Here's how the part is built. I have some questions about the finished solid (model axes, mm). Face numbers are marked on the shaded views. A direction names the side the tool comes from. Give positions to 0.01 mm unless a question says otherwise; leave off trailing zeros. Write each loop counter-clockwise with the first axis right and the second up, starting at its lowest first coordinate (ties: lowest second). Pieces come first, ordered by that corner, then holes. Notation, with made-up numbers: (83, 86) - (112, 86) arc R18 cw to (112, 90) - close; hole circle Ø8 at (40.5, 58). An arc over 180 degrees is marked (long way). Use a Markdown table: item, result.
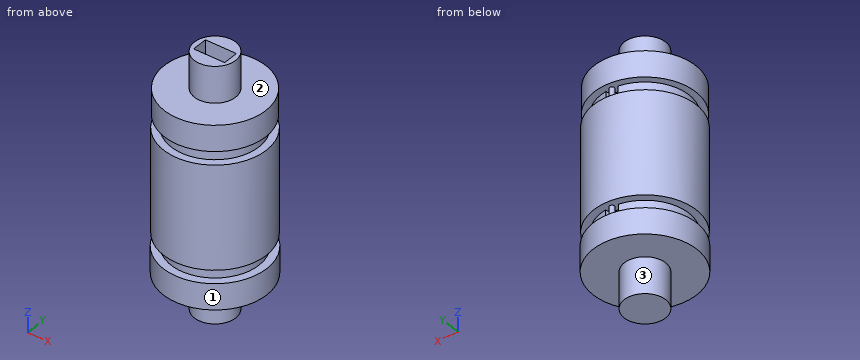
Autodesk Inventor part; units mm, degrees
ref_plane "YZ Plane" through (0, 0, 0) normal (1, 0, 0) x (0, 1, 0)
ref_plane "XZ Plane" through (0, 0, 0) normal (0, 1, 0) x (-1, 0, 0)
ref_plane "XY Plane" through (0, 0, 0) normal (0, 0, 1) x (1, 0, 0)
sketch "Sketch1" plane through (0, 0, 0) normal (0, 0, 1) x (1, 0, 0)
  circle A0 centre (0, 0) radius 10
  dimension "d0" = 20
extrude "Extrusion1" add sketch "Sketch1" along normal blind 5
sketch "Sketch2" plane through (0, 0, 5) normal (0, 0, 1) x (1, 0, 0)
  circle A0 centre (0, 0) radius 8.5
  circle A1 centre (-6.4588, 5.5258) radius 1.5
  dimension "d3" = 17
  dimension "d4" = 3
extrude "Extrusion2" add sketch "Sketch2" along normal blind 2.5 contours A0 A1 | A1 A0 picked at (2.8228, -1.7231) picked at (-6.0787, 5.1859)
sketch "Sketch3" plane through (0, 0, 7.5) normal (0, 0, 1) x (1, 0, 0)
  circle A0 centre (0, 0) radius 8.5
  circle A1 centre (0, 8.5) radius 1.25
  dimension "d7" = 2.5
extrude "Extrusion3" cut sketch "Sketch3" against normal blind 2.5 contours A1 A0 | A0 A1 picked at (0, 8.0765) picked at (0.0361, 8.9083)
sketch "Sketch4" plane through (0, 0, 7.5) normal (0, 0, 1) x (1, 0, 0)
  line L0 (-1.2337, 8.4081) -> (1.2466, 8.4081)
  circle A0 centre (0.0064, 8.4081) radius 0.5
  circle A1 centre (0, 0) radius 10
  dimension "d10" = 8.4081
  dimension "d11" = 1
extrude "Extrusion4" add sketch "Sketch4" against normal blind 2.5 contours A0 L0 | L0 A0
sketch "Sketch5" plane through (0, 0, 7.5) normal (0, 0, 1) x (1, 0, 0)
  circle A0 centre (0, 0) radius 9.9248
extrude "Extrusion5" add sketch "Sketch5" along normal blind 20
sketch "Sketch6" plane through (0, 0, 27.5) normal (0, 0, 1) x (1, 0, 0)
  circle A0 centre (0, 0) radius 8.5
extrude "Extrusion6" add sketch "Sketch6" along normal blind 2.5
sketch "Sketch7" plane through (0, 0, 30) normal (0, 0, 1) x (1, 0, 0)
  circle A0 centre (0.0064, 8.4081) radius 0.5
  circle A1 centre (0.0064, 8.4081) radius 0.5
  circle A2 centre (0.0064, 8.4081) radius 1.1746
  point P0 (0, 0)
extrude "Extrusion7" cut sketch "Sketch7" against normal blind 2.5 contours A0 | A2
sketch "Sketch8" plane through (0, 0, 30) normal (0, 0, 1) x (1, 0, 0)
  circle A0 centre (0.0064, 8.4081) radius 0.5
  circle A1 centre (0.0064, 8.4081) radius 0.5
  point P0 (0, 0)
extrude "Extrusion8" add sketch "Sketch8" against normal blind 2.5
sketch "Sketch9" plane through (0, 0, 30) normal (0, 0, 1) x (1, 0, 0)
  circle A0 centre (0, 0) radius 9.8132
extrude "Extrusion9" add sketch "Sketch9" along normal blind 5
sketch "Sketch10" plane through (0, 0, 35) normal (0, 0, 1) x (1, 0, 0)
  circle A0 centre (0, 0) radius 4
  line L0 (-3, 1.5) -> (3, 1.5)
  line L1 (3, 1.5) -> (3, -1.5)
  line L2 (3, -1.5) -> (-3, -1.5)
  line L3 (-3, -1.5) -> (-3, 1.5)
  dimension "d24" = 8
  dimension "d25" = 6
  dimension "d26" = 3
  dimension "d27" = 1.5
  dimension "d28" = 3
extrude "Extrusion10" add sketch "Sketch10" along normal blind 7
sketch "Sketch11" plane through (0, 0, 0) normal (0, 0, -1) x (-1, 0, 0)
  circle A0 centre (0, 0) radius 4
  dimension "d31" = 8
extrude "Extrusion11" add sketch "Sketch11" along normal blind 7
properties part number "Roller"
Item 1: For the marked faces 1, 2 and 3, which set-ups out of +Z, -Z, +X, -X, +Y, -Y let a thin tool reach every point of the face, with its end or its side?
Values:
| item | result |
|---|---|
| face 1 | +Z, -Z |
| face 2 | +Z |
| face 3 | -Z |
Item 2: If we section it at B-B, the plane z = 38: Write out the boundary of the cut face in (x, y).
Values:
| item | result |
|---|---|
| outline | circle Ø8 at (0, 0); hole (-3, -1.5) - (3, -1.5) - (3, 1.5) - (-3, 1.5) - close |
Item 3: Will these pins go through, and if not, where does the flat tip stop? pin 1 Ø4 at (x, z) = (-1.5, 36) entering from +Y; pin 2 Ø1.5 at (x, z) = (2.5, 33) entering from +Y; pin 3 Ø3.5 at (y, z) = (0.5, 38) entering from -X.
Values:
| item | result |
|---|---|
| pin 1 | stops at y = 9.81 |
| pin 2 | stops at y = 9.66 |
| pin 3 | stops at x = -4 |
Item 4: I need wall thicknesses on line 1 along Z through (x, y) = (-6.75, 6.75); line 2 along X through (y, z) = (-0.25, 28); line 3 along Z through (x, y) = (-4.25, -3). Which ranges of each line are inside material? Lowest first, please. Write a range as [from, to].
Values:
| item | result |
|---|---|
| line 1 | z = [0, 5], [7.5, 27.5], [30, 35] |
| line 2 | x = [-8.5, 8.5] |
| line 3 | z = [0, 35] |
Item 5: If we section it at D-D, the plane z = 24: Write out the boundary of the cut face in (x, y), plus the area to 3 significant figures.
Values:
| item | result |
|---|---|
| outline | circle Ø19.85 at (0, 0) |
| area | 309 mm2 |
Item 6: If we section it at C-C, the plane x = 5: Write out the boundary of the cut face in (y, z).
Values:
| item | result |
|---|---|
| outline | (-8.66, 0) - (8.66, 0) - (8.66, 5) - (6.87, 5) - (6.87, 7.5) - (8.57, 7.5) - (8.57, 27.5) - (6.87, 27.5) - (6.87, 30) - (8.44, 30) - (8.44, 35) - (-8.44, 35) - (-8.44, 30) - (-6.87, 30) - (-6.87, 27.5) - (-8.57, 27.5) - (-8.57, 7.5) - (-6.87, 7.5) - (-6.87, 5) - (-8.66, 5) - close |
